```python
from build123d import *

# Parameters (mm, degrees)
BOSS_EXTRUDE1_DEPTH = 3
SKETCH2_R           = 2.75
BOSS_EXTRUDE2_DEPTH = 2
BOSS_EXTRUDE2_TAPER = 48.36
SKETCH4_R           = 0.15
CUT_EXTRUDE1_DEPTH  = 1.5
SKETCH6_R           = 2.5
BOSS_EXTRUDE3_DEPTH = 6
SKETCH7_R           = 1
CUT_EXTRUDE3_DEPTH  = 9.5


with BuildPart() as part:
    # Sketch1 → Boss-Extrude1 (new body)
    with BuildSketch(Plane(origin=(0, 0, 0), x_dir=(1, 0, 0), z_dir=(0, 1, 0))):
        Polygon((4.041451884, 0), (2.020725942, 3.5), (-2.020725942, 3.5), (-4.041451884, 0), (-2.020725942, -3.5), (2.020725942, -3.5), align=None)
    extrude(amount=BOSS_EXTRUDE1_DEPTH)

    # Sketch2 → Boss-Extrude2 (add)
    with BuildSketch(Plane(origin=(0, 3, 0), x_dir=(1, 0, 0), z_dir=(0, 1, 0))):
        Circle(SKETCH2_R)
    extrude(amount=BOSS_EXTRUDE2_DEPTH, taper=BOSS_EXTRUDE2_TAPER)

    # Sketch4 → Cut-Extrude1 (cut)
    with BuildSketch(Plane(origin=(0, 5, 0), x_dir=(1, 0, 0), z_dir=(0, 1, 0))):
        with Locations(Location((0, 0, 0), (0, 0, 270))):
            Circle(SKETCH4_R)
    extrude(amount=-CUT_EXTRUDE1_DEPTH, mode=Mode.SUBTRACT)

    # Sketch6 → Boss-Extrude3 (add)
    with BuildSketch(Plane.XZ):
        with Locations(Location((0, 0, 0), (0, 0, 270))):
            Circle(SKETCH6_R)
    extrude(amount=BOSS_EXTRUDE3_DEPTH)

    # Sketch7 → Cut-Extrude3 (cut)
    with BuildSketch(Plane.XZ.offset(6)):
        with Locations(Location((0, 0, 0), (0, 0, 270))):
            Circle(SKETCH7_R)
    extrude(amount=-CUT_EXTRUDE3_DEPTH, mode=Mode.SUBTRACT)


solid = part.part
```
Here's how the part is built. I have some questions about the finished solid (model axes, mm). A direction names the side the tool comes from. Round coordinates to 2 decimals unless told otherwise and drop trailing zeros. Loops run counter-clockwise (first coordinate to the right, second up) from the corner with the lowest first, then second, coordinate; pieces in that order, holes last.
1. Suppose I cut it at A-A, the plane x = 0. Please give me the cut outline in (y, z), and give its area (3 significant figures).
Answers:
outline: (-6, -2.5) - (0, -2.5) - (0, -3.5) - (3, -3.5) - (3, -2.75) - (5, -0.5) - (5, -0.15) - (3.5, -0.15) - (3.5, -1) - (-6, -1) - close; (-6, 1) - (3.5, 1) - (3.5, 0.15) - (5, 0.15) - (5, 0.5) - (3, 2.75) - (3, 3.5) - (0, 3.5) - (0, 2.5) - (-6, 2.5) - close
area: 38.1 mm2
2. Suppose I cut it at D-D, the plane y = 3.75. Please give me the cut outline in (x, z), and give its area (3 significant figures).
Answers:
outline: circle Ø3.81 at (0, 0); hole circle Ø0.3 at (0, 0)
area: 11.3 mm2
3. If I drill on probe 1 along X at (y, z) = (-4, 0); probe 2 along Y at (x, z) = (2.25, -2); probe 3 along Z at (x, y) = (0.5, -2.5), over which ranges is the centre line in solid material (lowest first)?
Answers:
probe 1: x = -2.5 to -1, 1 to 2.5
probe 2: y = 0 to 3
probe 3: z = -2.45 to -0.87, 0.87 to 2.45
4. For faces 1 (the face through (1, 3, -3)), 2 (the face through (3, 0, 0)), 3 (the face through (0, 1, 3.5)), which set-ups out of +Z, -Z, +X, -X, +Y, -Y let a thin tool reach every point of the face, with its end or its side?
Answers:
face 1: +Y
face 2: -Y
face 3: +Z, +X, -X, +Y, -Y
5. Suppose I cut it at B-B, the plane y = 0.5. Please give me the cut outline in (x, z).
Answers:
outline: (-4.04, 0) - (-2.02, -3.5) - (2.02, -3.5) - (4.04, 0) - (2.02, 3.5) - (-2.02, 3.5) - close; hole circle Ø2 at (0, 0)
6. Suppose I cut it at C-C, the plane y = -2.75. Please give me the cut outline in (x, z).
Answers:
outline: circle Ø5 at (0, 0); hole circle Ø2 at (0, 0)
7. Thinking about a two-plate mould opening in Z: for faces 4 (the face through (-3, 1.5, -1.8)), 5 (the face through (-3.045, 1.479, 1.726)), 6 (the face through (0.24, 3.5, -0.21)), which applies, released by +Z, released by -Z, zero draft, split by the parting line, or undercut?
Answers:
face 4: released by -Z
face 5: released by +Z
face 6: undercut
8. Will this pin go through, and if not, where does the flat tip stop? pin 1 (2 mm diameter, centred on x = 0.5, z = 0, fed in from -Y).
Answers:
pin 1: stops at y = -6
